Can you work these out from the model? Positions are in its coordinate system, mm. A direction names the side the tool comes from. Round coordinates to 2 decimals unless told otherwise and drop trailing zeros. Loops run counter-clockwise (first coordinate to the right, second up) from the corner with the lowest first, then second, coordinate; pieces in that order, holes last.
```python
from build123d import *

# Parameters (mm, degrees)
BOSS_EXTRUDE1_DEPTH     = 3
BOSS_EXTRUDE2_DEPTH     = 12
BOSS_EXTRUDE3_DEPTH     = 4.17
CUT_EXTRUDE1_DEPTH      = 101.179165
CUT_EXTRUDE1_DEPTH_BACK = 101.179165
SKETCH3_R               = 2
CHAMFER1_SIZE           = 6
SKETCH8_R               = 4
CUT_EXTRUDE2_DEPTH      = 7.17
CHAMFER2_SIZE           = 1
CUT_EXTRUDE4_START      = -5
SKETCH9_R               = 4
CUT_EXTRUDE4_DEPTH      = 5
CHAMFER3_SIZE           = 2


with BuildPart() as part:
    # Sketch1 → Boss-Extrude1 (new body)
    with BuildSketch(Plane(origin=(0, 0, 0), x_dir=(1, 0, 0), z_dir=(0, 1, 0))):
        Polygon((-95.41, 0), (95.41, 0), (69.5, 25.91), (-69.5, 25.91), align=None)
    extrude(amount=BOSS_EXTRUDE1_DEPTH)

    # Sketch5 → Boss-Extrude2 (add)
    with BuildSketch(Plane(origin=(0, 3, 0), x_dir=(1, 0, 0), z_dir=(0, 1, 0))):
        with BuildLine():
            Line((-64.496944889, 25.91), (-69.5, 25.91))
            Line((-69.5, 25.91), (-95.41, 0))
            Line((-95.41, 0), (95.41, 0))
            Line((95.41, 0), (69.5, 25.91))
            Line((69.5, 25.91), (64.496944889, 25.91))
            ThreePointArc((64.496944889, 25.91), (54.829686624, 24.966540009), (45.527255216, 22.171764706))
            ThreePointArc((45.527255216, 22.171764706), (0, 13.2), (-45.527255216, 22.171764706))
            ThreePointArc((-45.527255216, 22.171764706), (-54.829686624, 24.966540009), (-64.496944889, 25.91))
        make_face()
    extrude(amount=BOSS_EXTRUDE2_DEPTH)

    # Sketch7 → Boss-Extrude3 (add)
    with BuildSketch(Plane(origin=(0, 15, 0), x_dir=(1, 0, 0), z_dir=(0, 1, 0))):
        Polygon((-95.41, 0), (-69.5, 25.91), (69.5, 25.91), (95.41, 0), align=None)
    extrude(amount=BOSS_EXTRUDE3_DEPTH)

    # Sketch3 → Cut-Extrude1 (cut, two sides: drawn at the far end of the back side and taken through both)
    with BuildSketch(Plane(origin=(0, 3, 0), x_dir=(1, 0, 0), z_dir=(0, 1, 0)).offset(-CUT_EXTRUDE1_DEPTH_BACK)):
        with Locations(Location((-60, 12, 0), (0, 0, 270))):
            Circle(SKETCH3_R)
        with Locations(Location((60, 12, 0), (0, 0, 90))):
            Circle(SKETCH3_R)
    extrude(amount=CUT_EXTRUDE1_DEPTH + CUT_EXTRUDE1_DEPTH_BACK, mode=Mode.SUBTRACT)

    # Chamfer1
    chamfer1_edges = [part.edges().sort_by_distance(p)[0] for p in [
        (0, 19.17, 0),
    ]]
    chamfer(chamfer1_edges, length=CHAMFER1_SIZE)

    # Sketch8 → Cut-Extrude2 (cut)
    with BuildSketch(Plane(origin=(0, 19.17, 0), x_dir=(1, 0, 0), z_dir=(0, 1, 0))):
        with Locations(Location((-60, 12, 0), (0, 0, 270))):
            Circle(SKETCH8_R)
        with Locations(Location((60, 12, 0), (0, 0, 270))):
            Circle(SKETCH8_R)
    extrude(amount=-CUT_EXTRUDE2_DEPTH, mode=Mode.SUBTRACT)

    # Chamfer2
    chamfer2_edges = [part.edges().sort_by_distance(p)[0] for p in [
        (-60, 19.17, -16),
        (60, 19.17, -16),
    ]]
    chamfer(chamfer2_edges, length=CHAMFER2_SIZE)

    # Sketch9 → Cut-Extrude4 (cut)
    with BuildSketch(Plane(origin=(0, 0, 0), x_dir=(-1, 0, 0), z_dir=(0, -1, 0)).offset(CUT_EXTRUDE4_START)):
        with Locations(Location((60, 12, 0), (0, 0, 270))):
            Circle(SKETCH9_R)
        with Locations(Location((30, 12, 0), (0, 0, 90))):
            Circle(SKETCH9_R)
        with Locations(Location((-30, 12, 0), (0, 0, 90))):
            Circle(SKETCH9_R)
        with Locations(Location((-60, 12, 0), (0, 0, 270))):
            Circle(SKETCH9_R)
    extrude(amount=CUT_EXTRUDE4_DEPTH, mode=Mode.SUBTRACT)

    # Chamfer3
    chamfer3_edges = [part.edges().sort_by_distance(p)[0] for p in [
        (0, 19.17, -25.91),
    ]]
    chamfer(chamfer3_edges, length=CHAMFER3_SIZE)


solid = part.part
```
(1) Suppose I cut it at B-B (x = 60). Write out the boundary of the cut face in (y, z), then the cut area to 3 significant figures.
(2) If I drill on line 1 (Y direction, x = -29, z = -19.5); line 2 (X direction, y = 3.75, z = -12); line 3 (X direction, y = 14.5, z = -10.75), over which ranges is the centre line in solid material (lowest first)?
(3) Suppose I cut it at A-A (y = 8.75). Write out the boundary of the cut face in (x, z), then the cut area to 3 significant figures.
(4) We'd pull the mould along X, two halves only. Please class faces 1 (the flat face through (-82.64, 9.45, -12.77)), 2 (the cylindrical face through (-55, 9, -25)), 3 (the flat face through (82.27, 9.45, -13.14)): released by +X, released by -X, zero draft, split by the parting line, or undercut.
(5) Suppose I cut it at C-C (z = -3.25). Write out the boundary of the cut face in (x, y), then the cut area to 3 significant figures.
(6) Which directions (+Z, -Z, +X, -X, +Y, -Y) give clear straight access to the entire face, cutting with the end or side of a thin tool? Please do faces 4 (the cylindrical face through (55, 9, -25)), 5 (the cylindrical face through (33.966, 2.535, -11.479)), 6 (the cylindrical face through (-63.905, 15.128, -12.867)).
(7) Suppose I cut it at D-D (x = 30). Write out the boundary of the cut face in (y, z).
(8) For pin 1 (7 mm diameter, centred on x = 30, z = -12, fed in from -Y); pin 2 (9 mm diameter, centred on x = -60, z = -12, fed in from +Y); pin 3 (2.5 mm diameter, centred on x = 60, z = -12, fed in from +Y); pin 4 (6 mm diameter, centred on y = 4.5, z = -22.5, fed in from +X), each with a flat end and sliding along its axis, tell me the tip position at first contact or that it passes through.
Check result:
1. outline: (0, -25.91) - (3, -25.91) - (3, -25.71) - (15, -25.71) - (15, -25.91) - (17.17, -25.91) - (19.17, -23.91) - (19.17, -17) - (18.17, -16) - (12, -16) - (12, -14) - (5, -14) - (5, -16) - (0, -16) - close; (0, -8) - (5, -8) - (5, -10) - (12, -10) - (12, -8) - (18.17, -8) - (19.17, -7) - (19.17, -6) - (13.17, 0) - (0, 0) - close
1. area: 348 mm2
2. line 1: y = 0 to 3, 15 to 19.17
2. line 2: x = -83.41 to -64, -56 to -34, -26 to 26, 34 to 56, 64 to 83.41
2. line 3: x = -84.66 to -63.8, -56.2 to 56.2, 63.8 to 84.66
3. outline: (-95.41, 0) - (-69.5, -25.91) - (-64.5, -25.91) arc R50 ccw to (-45.53, -22.17) arc R120 cw to (45.53, -22.17) arc R50 ccw to (64.5, -25.91) - (69.5, -25.91) - (95.41, 0) - close; hole circle Ø4 at (-60, -12); hole circle Ø4 at (60, -12)
3. area: 3,310 mm2
4. face 1: released by -X
4. face 2: undercut
4. face 3: released by +X
5. outline: (-92.16, 0) - (92.16, 0) - (92.16, 16.42) - (-92.16, 16.42) - close
5. area: 3,030 mm2
6. face 4: -Z
6. face 5: -Y
6. face 6: +Y
7. outline: (0, -25.91) - (3, -25.91) - (3, -17.01) - (15, -17.01) - (15, -25.91) - (17.17, -25.91) - (19.17, -23.91) - (19.17, -6) - (13.17, 0) - (0, 0) - (0, -8) - (5, -8) - (5, -16) - (0, -16) - close
8. pin 1: stops at y = 5
8. pin 2: stops at y = 18.67
8. pin 3: passes through
8. pin 4: stops at x = 75.91
